from build123d import *

# Parameters (mm, degrees)
F0_W     = 25
F0_H     = 75
F1_DEPTH = 50
F2_W     = 50
F2_H     = 50
F3_DEPTH = 17.5
F4_W     = 35
F4_H     = 50
F5_DEPTH = 30
F6_W     = 15
F6_H     = 50
F6_W_2   = 35
F7_DEPTH = 25
F8_W     = 40
F8_H     = 50
F8_H_2   = 25
F9_DEPTH = 10


with BuildPart() as f1:
    # F0 (on Front) → F1 (new body)
    with BuildSketch(Plane.XZ):
        with Locations((12.5, 37.5)):
            Rectangle(F0_W, F0_H)
    extrude(amount=F1_DEPTH)

    # F2 (on face) → F3 (join)
    with BuildSketch(Plane.YZ.offset(25)):
        with Locations((-25, 25)):
            Rectangle(F2_W, F2_H)
    extrude(amount=F3_DEPTH)

    # F4 (on face) → F5 (join)
    with BuildSketch(Plane.YZ.offset(42.5)):
        with Locations((-17.5, 25)):
            Rectangle(F4_W, F4_H)
    extrude(amount=F5_DEPTH)

    # F6 (on face) → F7 (join)
    with BuildSketch(Plane.YZ.offset(72.5)):
        with Locations((-42.5, 25)):
            Rectangle(F6_W, F6_H)
        with Locations((-17.5, 25)):
            Rectangle(F6_W_2, F6_H)
    extrude(amount=F7_DEPTH)

    # F8 (on face) → F9 (join)
    with BuildSketch(Plane.YZ.offset(97.5)):
        with Locations((-20, 25)):
            Rectangle(F8_W, F8_H)
        with Locations((-20, 62.5)):
            Rectangle(F8_W, F8_H_2)
    extrude(amount=F9_DEPTH)


solid = f1.part
Read the model definition and answer for the solid it produces. Units are mm, in the model's axes. A direction names the side the tool comes from. Coordinates: 2 decimals unless noted, no trailing zeros. Loops run counter-clockwise (first coordinate to the right, second up) from the corner with the lowest first, then second, coordinate; pieces in that order, holes last. Notation, with made-up numbers: (-31, 49.25) -> (1, 49.25) arc R19 cw to (1, 57.25) -> close; hole circle Ø5 at (-1, 59). An arc over 180 degrees is marked (long way). Write item = value, one per line. Start each with the question number.
1) Given P1, Ø15, axis at x = 58, z = 14, coming from the -Y side; P2, Ø5, axis at x = 82.5, y = -27, coming from the +Z side; P3, Ø11, axis at x = 104.5, z = 29.5, coming from the -Y side, each flat-ended and moving along its own axis, determine where each tip first touches the part or whether it passes through.
2) The mould has two halves that part along X. Classify faces 4 (the face through (85, -50, 25)), 5 (the face through (97.5, -20, 63)), 6 (the face through (97.5, -45, 25)): pulls with the +X half, pulls with the -X half, needs draft (parallel to the pull), parting line crosses it, or undercut.
3) The part is cut by section B-B, the plane y = -7.5. Determine the outline of the cut face in (x, z).
4) The part is cut by section D-D, the plane x = 99.5. Determine the outline of the cut face in (y, z), plus the area to 3 significant figures.
5) For faces 1 (the face through (57, -35, 25)), 2 (the face through (61, -19, 50)), 3 (the face through (102, -40, 38)), determine the directions among +Z, -Z, +X, -X, +Y, -Y from which every point of the face is accessible in a straight line to the end or side of a thin tool.
6) The part is cut by section A-A, the plane z = 17. Determine the outline of the cut face in (x, y), plus the area to 4 significant figures.
7) Find the intervals of material crossed by L1, parallel to X at y = -39, z = 65.5; L2, parallel to X at y = -40.5, z = 10.5; L3, parallel to Z at x = 28, y = -17, in increasing order. Write a range as from..to.
8) The part is cut by section C-C, the plane x = 56. Determine the outline of the cut face in (y, z), plus the area to 3 significant figures.
Result:
q1.P1 = -35
q1.P2 = 50
q1.P3 = -40
q2.face_4 = needs draft
q2.face_5 = undercut
q2.face_6 = pulls with the +X half
q3.outline = (0, 0) -> (107.5, 0) -> (107.5, 75) -> (97.5, 75) -> (97.5, 50) -> (25, 50) -> (25, 75) -> (0, 75) -> close
q4.outline = (-40, 0) -> (0, 0) -> (0, 75) -> (-40, 75) -> close
q4.area = 3,000 mm²
q5.face_1 = +Z, -Z, -Y
q5.face_2 = +Z, +Y, -Y
q5.face_3 = +Z, -Z, +X, -Y
q6.outline = (0, -50) -> (42.5, -50) -> (42.5, -35) -> (72.5, -35) -> (72.5, -50) -> (97.5, -50) -> (97.5, -40) -> (107.5, -40) -> (107.5, 0) -> (0, 0) -> close
q6.area = 4,825 mm²
q7.L1 = 0..25, 97.5..107.5
q7.L2 = 0..42.5, 72.5..97.5
q7.L3 = 0..50
q8.outline = (-35, 0) -> (0, 0) -> (0, 50) -> (-35, 50) -> close
q8.area = 1,750 mm²
